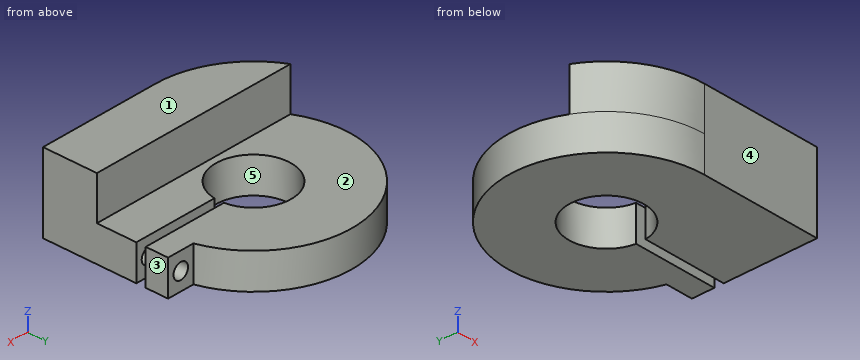
```python
from build123d import *
from build123d.topology import SkipClean

# Parameters (mm, degrees)
BOSS_EXTRUDE1_DEPTH = 4.5
BOSS_EXTRUDE2_DEPTH = 5.5
SKETCH4_R           = 1
CUT_EXTRUDE1_DEPTH  = 5.5


with BuildPart() as part:
    # Sketch1 → Boss-Extrude1 (new body)
    with BuildSketch(Plane.XY):
        with BuildLine():
            Line((0, -12.5), (15.5, -12.5))
            Line((15.5, -12.5), (15.5, -0.6))
            Line((15.5, -0.6), (4.735951007, -0.6))
            ThreePointArc((4.735951007, -0.6), (-4.77380686, 0), (4.735951007, 0.6))
            Line((4.735951007, 0.6), (15.5, 0.6))
            Line((15.5, 0.6), (15.5, 3.452502188))
            Line((15.5, 3.452502188), (12.013751647, 3.452502188))
            ThreePointArc((12.013751647, 3.452502188), (-9.985145901, 7.519764712), (0, -12.5))
        make_face()
    extrude(amount=BOSS_EXTRUDE1_DEPTH)

    # Sketch2 → Boss-Extrude2 (add)
    with SkipClean():  # the faces are left unmerged after this step: merging them gives an invalid solid
        with BuildSketch(Plane.XY.offset(4.5)):
            with BuildLine():
                Line((15.5, -12.5), (0, -12.5))
                ThreePointArc((0, -12.5), (-6.553255279, -10.644474869), (-11.160953781, -5.628775239))
                Line((-11.160953781, -5.628775239), (15.5, -5.628775239))
                Line((15.5, -5.628775239), (15.5, -12.5))
            make_face()
        extrude(amount=BOSS_EXTRUDE2_DEPTH)

    # Sketch4 → Cut-Extrude1 (cut)
    with SkipClean():  # the faces are left unmerged after this step: merging them gives an invalid solid
        with BuildSketch(Plane(origin=(0, 3.452502188, 0), x_dir=(1, 0, 0), z_dir=(0, 1, 0))):
            with Locations(Location((13.756875824, -2.25, 0), (0, 0, 180))):
                Circle(SKETCH4_R)
        extrude(amount=-CUT_EXTRUDE1_DEPTH, mode=Mode.SUBTRACT)


solid = part.part
```
Design review of the part built by this model. Coordinates are the model's own, in mm. Face numbers are marked on the shaded views. A direction names the side the tool comes from. Give positions to 0.01 mm unless a question says otherwise; leave off trailing zeros. Loops run counter-clockwise (first coordinate to the right, second up) from the corner with the lowest first, then second, coordinate; pieces in that order, holes last. Notation, with made-up numbers: M 49.25,-19.75 L 61.25,-19.75 A23 ccw 61.25,-9.75 Z; hole C -15,86.5 d10. An arc over 180 degrees is marked long. Return JSON: item names as keys, results as strings. Group by question number.
Item 1: Tool access review of the marked faces 1 and 2: name each direction out of +Z, -Z, +X, -X, +Y, -Y from which nothing blocks a thin tool from reaching the whole face with its end or side.
Item 2: We need section A-A (z = 2.25). Give the boundary of the cut face in (x, y), and give its area (3 significant figures).
Item 3: Insertion check: pin 1 Ø3 at (y, z) = (6.5, 4) entering from -X; pin 2 Ø1.3 at (x, z) = (9, 2.5) entering from +Y; pin 3 Ø2 at (y, z) = (1.5, 5) entering from -X; pin 4 Ø8.5 at (x, y) = (0, 0) entering from +Z. Each pin has a flat end and moves straight along its axis. Give the tip position at first contact, or say it passes through.
Item 4: Mouldability with a two-part tool opening along X and no side actions: class the marked faces 3, 4 and 5 as released by +X, released by -X, zero draft, split by the parting line, or undercut.
Item 5: For probe 1 along Y at (x, z) = (0, 3.35); probe 2 along Z at (x, y) = (-11, -1); probe 3 along X at (y, z) = (1.25, 2.75), list the stretches that pass through material, from the lowest coordinate up.
Item 6: We need section B-B (x = 9.75). Give the boundary of the cut face in (y, z).
Item 7: We need section C-C (y = -2.5). Give the boundary of the cut face in (x, z), and give its area (3 significant figures).
Item 8: We need section D-D (x = -10.5). Give the boundary of the cut face in (y, z).
Output:
{
 "1": {"face 1": "+Z, +X, -X, +Y, -Y", "face 2": "+Z, +X, -X, +Y"},
 "2": {"outline": "M 0,-12.5 L 15.5,-12.5 L 15.5,-0.6 L 14.76,-0.6 L 14.76,-2.05 L 12.76,-2.05 L 12.76,-0.6 L 4.74,-0.6 A4.77 cw long 4.74,0.6 L 12.76,0.6 L 12.76,3.45 L 12.01,3.45 A12.5 ccw long Z; M 14.76,0.6 L 15.5,0.6 L 15.5,3.45 L 14.76,3.45 Z", "area": "480 mm^2"},
 "3": {"pin 1": "stops at x = -11.46", "pin 2": "stops at y = 9.3", "pin 3": "stops at x = -12.48", "pin 4": "passes through"},
 "4": {"face 3": "released by +X", "face 4": "zero draft", "face 5": "undercut"},
 "5": {"probe 1": "y = -12.5 to -4.77, 4.77 to 12.5", "probe 2": "z = 0 to 4.5", "probe 3": "x = -12.44 to -4.61, 4.61 to 12.89, 14.62 to 15.5"},
 "6": {"outline": "M -12.5,0 L -0.6,0 L -0.6,4.5 L -5.63,4.5 L -5.63,10 L -12.5,10 Z; M 0.6,0 L 7.82,0 L 7.82,4.5 L 0.6,4.5 Z"},
 "7": {"outline": "M -12.25,0 L -4.07,0 L -4.07,4.5 L -12.25,4.5 Z; M 4.07,0 L 15.5,0 L 15.5,4.5 L 4.07,4.5 Z", "area": "88.3 mm^2"},
 "8": {"outline": "M -6.78,0 L 6.78,0 L 6.78,4.5 L -5.63,4.5 L -5.63,10 L -6.78,10 Z"}
}
